Verification items for this drawing (mm, ordinates from the low corner). A direction names the side the tool comes from. Coordinates: 2 decimals unless noted, no trailing zeros. Order: outer loops, then holes, each group sorted by start corner. A loop starts at its lowest first (then second) coordinate and runs counter-clockwise, first axis right, second up. Notation, with made-up numbers: M 20.5,3 L 39.5,3 A11 cw 39.5,21 Z; hole C 39,3.5 d11. An arc over 180 degrees is marked long. One line per item, written item: value. Start each with the question number.
1) Sectioned sample at A-A, the plane y = 15. Enter the section's corners in (x, z), then the cut area to 3 significant figures.
2) Sectioned sample at C-C, the plane x = 90. Enter the section's corners in (y, z), then the cut area to 3 significant figures.
3) Sectioned sample at B-B, the plane z = 90. Enter the section's corners in (x, y), then the cut area to 3 significant figures.
4) Access from +Z, -Z, +X, -X, +Y, -Y to the whole of each face (thin tool, end or side, straight path). Record for the marked faces 1, 2 and 3.
5) Thickness scan on L1, parallel to Z at x = 4, y = 15; L2, parallel to Y at x = 90, z = 3.25; L3, parallel to Z at x = 83, y = 20. Record the ranges inside material, lowest first. Write a range as from..to.
6) Go/stop test with flat-tipped pins: P1, Ø1, axis at x = 50.5, y = 16.5, coming from the +Z side; P2, Ø4, axis at x = 82.5, y = 16.5, coming from the +Z side; P3, Ø10, axis at y = 14, z = 94.5, coming from the +X side. Record where each tip stops, or that it passes through.
7) Sectioned sample at D-D, the plane z = 35. Enter the section's corners in (x, y).
8) Draft check along X on the marked faces 4, 5, 6 and 7. Enter one of: pulls with the +X half, pulls with the -X half, needs draft (parallel to the pull), parting line crosses it, or undercut.
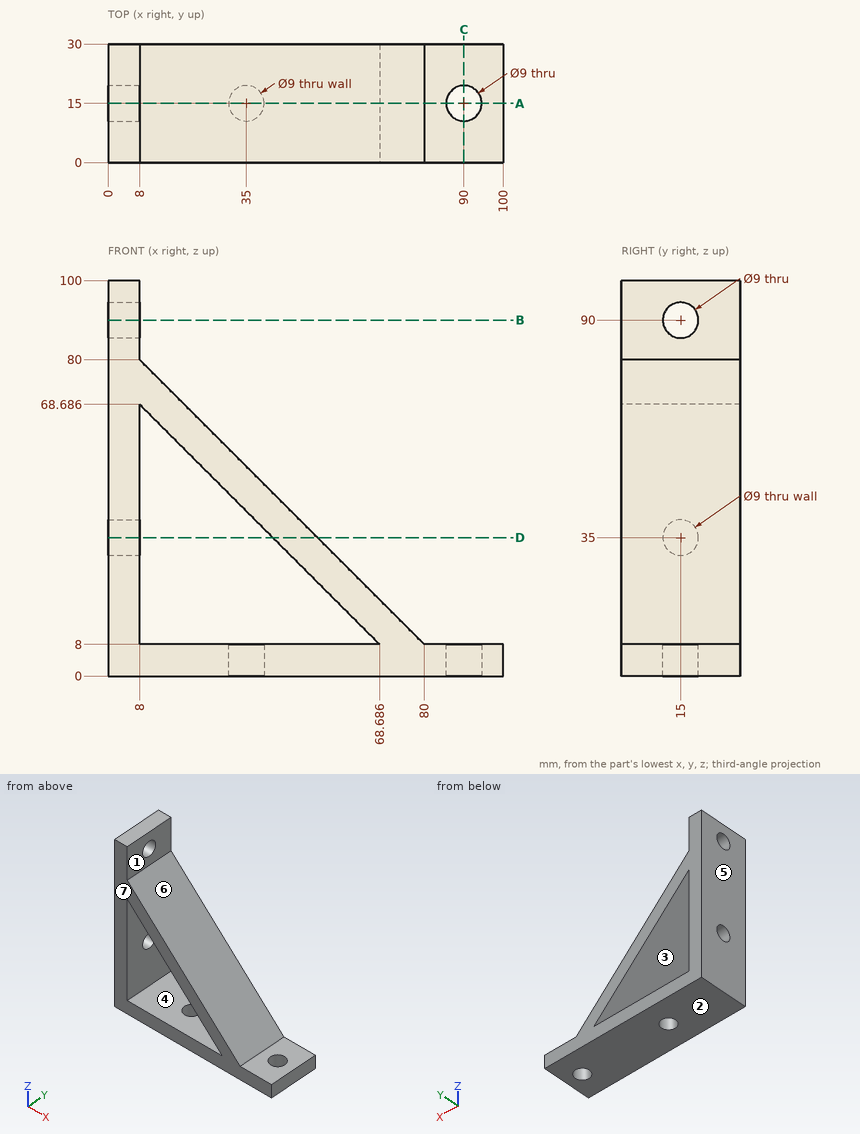
Final values:
1. outline: M 0,0 L 30.5,0 L 30.5,8 L 8,8 L 8,30.5 L 0,30.5 Z; M 0,39.5 L 8,39.5 L 8,68.69 L 68.69,8 L 39.5,8 L 39.5,0 L 85.5,0 L 85.5,8 L 80,8 L 8,80 L 8,85.5 L 0,85.5 Z; M 0,94.5 L 8,94.5 L 8,100 L 0,100 Z; M 94.5,0 L 100,0 L 100,8 L 94.5,8 Z
1. area: 2,000 mm^2
2. outline: M 0,0 L 10.5,0 L 10.5,8 L 0,8 Z; M 19.5,0 L 30,0 L 30,8 L 19.5,8 Z
2. area: 168 mm^2
3. outline: M 0,0 L 8,0 L 8,10.5 L 0,10.5 Z; M 0,19.5 L 8,19.5 L 8,30 L 0,30 Z
3. area: 168 mm^2
4. face 1: +Z, +X, +Y, -Y
4. face 2: -Z, +X, -X, +Y, -Y
4. face 3: +Y, -Y
5. L1: z = 0..30.5, 39.5..85.5, 94.5..100
5. L2: y = 0..10.5, 19.5..30
5. L3: z = 0..8
6. P1: stops at z = 38
6. P2: stops at z = 8
6. P3: stops at x = 8
7. outline: M 0,0 L 8,0 L 8,10.5 L 0,10.5 Z; M 0,19.5 L 8,19.5 L 8,30 L 0,30 Z; M 41.69,0 L 53,0 L 53,30 L 41.69,30 Z
8. face 4: undercut
8. face 5: pulls with the -X half
8. face 6: pulls with the +X half
8. face 7: needs draft
